Work out the finished part from the listing and answer in its coordinate system (mm). Give positions to 0.01 mm unless a question says otherwise; leave off trailing zeros. Order: outer loops, then holes, each group sorted by start corner. A loop starts at its lowest first (then second) coordinate and runs counter-clockwise, first axis right, second up. Notation, with made-up numbers: (-6.75, 71) - (9.25, 71) arc R17 cw to (9.25, 86) - close; hole circle Ø11 at (61.5, 40). An arc over 180 degrees is marked (long way). Return JSON: item names as keys, results as strings. Group by question number.
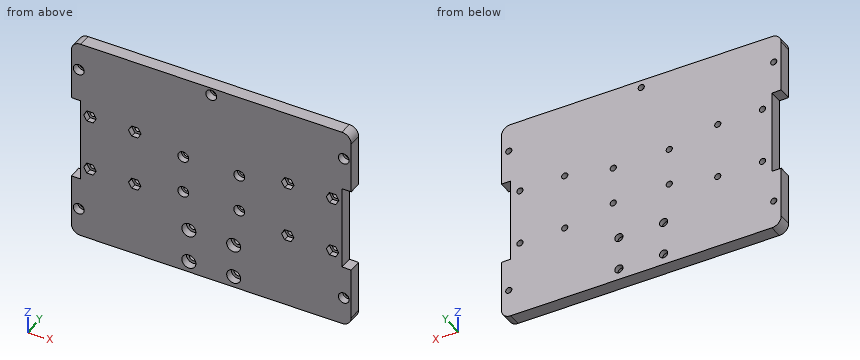
from build123d import *

# Parameters (mm, degrees)
SKETCH_1_W          = 150
SKETCH_1_H          = 110
EXTRUDE_1_DEPTH     = 7
FILLET_1_R          = 5
SKETCH_2_R          = 1.65
SKETCH_2_R_2        = 2.2
CUT_EXTRUDE_1_DEPTH = 8
SKETCH_5_R          = 3.75
CUT_EXTRUDE_3_DEPTH = 4.2
CUT_EXTRUDE_4_DEPTH = 3
SKETCH_7_R          = 2.9
CUT_EXTRUDE_5_DEPTH = 3.3
SKETCH_8_R          = 1.65
CUT_EXTRUDE_6_DEPTH = 8
SKETCH_9_R          = 2.9
CUT_EXTRUDE_7_DEPTH = 4
SKETCH_10_W         = 5
SKETCH_10_H         = 45
CUT_EXTRUDE_8_DEPTH = 8


with BuildPart() as part:
    # 草图1 → 凸台-拉伸1 (new body)
    with BuildSketch(Plane(origin=(0, 0, 0), x_dir=(1, 0, 0), z_dir=(0, 1, 0))):
        Rectangle(SKETCH_1_W, SKETCH_1_H)
    extrude(amount=EXTRUDE_1_DEPTH)

    # 圆角1
    fillet_1_edges = [part.edges().sort_by_distance(p)[0] for p in [
        (75, 3.5, 55),
        (-75, 3.5, 55),
        (-75, 3.5, -55),
        (75, 3.5, -55),
    ]]
    fillet(fillet_1_edges, radius=FILLET_1_R)

    # 草图2 → 切除-拉伸1 (cut, through all)
    with BuildSketch(Plane(origin=(0, 7, 0), x_dir=(1, 0, 0), z_dir=(0, 1, 0))):
        with Locations((65, -15)):
            Circle(SKETCH_2_R)
        with Locations((41, -15)):
            Circle(SKETCH_2_R)
        with Locations((41, 15)):
            Circle(SKETCH_2_R)
        with Locations((65, 15)):
            Circle(SKETCH_2_R)
        with Locations((-65, 15)):
            Circle(SKETCH_2_R)
        with Locations((-41, 15)):
            Circle(SKETCH_2_R)
        with Locations((-41, -15)):
            Circle(SKETCH_2_R)
        with Locations((-65, -15)):
            Circle(SKETCH_2_R)
        with Locations((12, 31)):
            Circle(SKETCH_2_R_2)
        with Locations((12, 49)):
            Circle(SKETCH_2_R_2)
        with Locations((-12, 49)):
            Circle(SKETCH_2_R_2)
        with Locations((-12, 31)):
            Circle(SKETCH_2_R_2)
        with Locations((15, 10)):
            Circle(SKETCH_2_R)
        with Locations((15, -10)):
            Circle(SKETCH_2_R)
        with Locations((-15, -10)):
            Circle(SKETCH_2_R)
        with Locations((-15, 10)):
            Circle(SKETCH_2_R)
    extrude(amount=-CUT_EXTRUDE_1_DEPTH, mode=Mode.SUBTRACT)

    # 草图5 → 切除-拉伸3 (cut)
    with BuildSketch(Plane.XZ):
        with Locations((12, -49)):
            Circle(SKETCH_5_R)
        with Locations((12, -31)):
            Circle(SKETCH_5_R)
        with Locations((-12, -31)):
            Circle(SKETCH_5_R)
        with Locations((-12, -49)):
            Circle(SKETCH_5_R)
    extrude(amount=-CUT_EXTRUDE_3_DEPTH, mode=Mode.SUBTRACT)

    # 草图6 → 切除-拉伸4 (cut)
    with BuildSketch(Plane.XZ):
        Polygon((-39.325684219, 17.9), (-37.651368439, 15), (-39.325684219, 12.1), (-42.674315781, 12.1), (-44.348631561, 15), (-42.674315781, 17.9), align=None)
        Polygon((61.651368439, -15), (63.325684219, -17.9), (66.674315781, -17.9), (68.348631561, -15), (66.674315781, -12.1), (63.325684219, -12.1), align=None)
        Polygon((37.651368439, -15), (39.325684219, -17.9), (42.674315781, -17.9), (44.348631561, -15), (42.674315781, -12.1), (39.325684219, -12.1), align=None)
        Polygon((61.651368439, 15), (63.325684219, 12.1), (66.674315781, 12.1), (68.348631561, 15), (66.674315781, 17.9), (63.325684219, 17.9), align=None)
        Polygon((37.651368439, 15), (39.325684219, 12.1), (42.674315781, 12.1), (44.348631561, 15), (42.674315781, 17.9), (39.325684219, 17.9), align=None)
        Polygon((-63.325684219, 17.9), (-61.651368439, 15), (-63.325684219, 12.1), (-66.674315781, 12.1), (-68.348631561, 15), (-66.674315781, 17.9), align=None)
        Polygon((-39.325684219, -12.1), (-37.651368439, -15), (-39.325684219, -17.9), (-42.674315781, -17.9), (-44.348631561, -15), (-42.674315781, -12.1), align=None)
        Polygon((-63.325684219, -12.1), (-61.651368439, -15), (-63.325684219, -17.9), (-66.674315781, -17.9), (-68.348631561, -15), (-66.674315781, -12.1), align=None)
    extrude(amount=-CUT_EXTRUDE_4_DEPTH, mode=Mode.SUBTRACT)

    # 草图7 → 切除-拉伸5 (cut)
    with BuildSketch(Plane.XZ):
        with Locations((15, -10)):
            Circle(SKETCH_7_R)
        with Locations((15, 10)):
            Circle(SKETCH_7_R)
        with Locations((-15, 10)):
            Circle(SKETCH_7_R)
        with Locations((-15, -10)):
            Circle(SKETCH_7_R)
    extrude(amount=-CUT_EXTRUDE_5_DEPTH, mode=Mode.SUBTRACT)

    # 草图8 → 切除-拉伸6 (cut, through all)
    with BuildSketch(Plane.XZ):
        with Locations((71, 40)):
            Circle(SKETCH_8_R)
        with Locations((71, -40)):
            Circle(SKETCH_8_R)
        with Locations((-71, -40)):
            Circle(SKETCH_8_R)
        with Locations((-71, 40)):
            Circle(SKETCH_8_R)
        with Locations((0, 51)):
            Circle(SKETCH_8_R)
    extrude(amount=-CUT_EXTRUDE_6_DEPTH, mode=Mode.SUBTRACT)

    # 草图9 → 切除-拉伸7 (cut)
    with BuildSketch(Plane.XZ):
        with Locations((71, 40)):
            Circle(SKETCH_9_R)
        with Locations((71, -40)):
            Circle(SKETCH_9_R)
        with Locations((-71, 40)):
            Circle(SKETCH_9_R)
        with Locations((-71, -40)):
            Circle(SKETCH_9_R)
        with Locations((0, 51)):
            Circle(SKETCH_9_R)
    extrude(amount=-CUT_EXTRUDE_7_DEPTH, mode=Mode.SUBTRACT)

    # 草图10 → 切除-拉伸8 (cut, through all)
    with BuildSketch(Plane(origin=(0, 7, 0), x_dir=(1, 0, 0), z_dir=(0, 1, 0))):
        with Locations((72.5, 0)):
            Rectangle(SKETCH_10_W, SKETCH_10_H)
        with Locations((-72.5, 0)):
            Rectangle(SKETCH_10_W, SKETCH_10_H)
    extrude(amount=-CUT_EXTRUDE_8_DEPTH, mode=Mode.SUBTRACT)


solid = part.part
1. The part is cut by section B-B (x = 0). Give the vertices of the cut face in (y, z), and give its area (3 significant figures).
2. The part is cut by section C-C (y = 1.5). State how many separate pieces and enclosed holes the cut face has, and give its area (3 significant figures).
3. The part is cut by section A-A (x = 41). Give the vertices of the cut face in (y, z), and give its area (3 significant figures).
4. Consider probe 1 along Z at (x, y) = (-64.5, 1.75); probe 2 along X at (y, z) = (5.75, -31); probe 3 along Z at (x, y) = (-12, 5.95). Determine where each line is inside the solid, lowest interval first. Write a range as from..to.
5. Each of these flat-tipped pins is pushed along its axis until it touches: pin 1 (6 mm diameter, centred on x = 12, z = -49, fed in from -Y); pin 2 (4.5 mm diameter, centred on x = 65.5, z = -15, fed in from -Y); pin 3 (3.5 mm diameter, centred on x = 71, z = 40, fed in from -Y). Where does it stop, or does it pass through?
Answers:
{
 "1": {"outline": "(0, -55) - (7, -55) - (7, 49.35) - (4, 49.35) - (4, 48.1) - (0, 48.1) - close; (0, 53.9) - (4, 53.9) - (4, 52.65) - (7, 52.65) - (7, 55) - (0, 55) - close", "area": "737 mm^2"},
 "2": {"separate pieces": "1", "enclosed holes": "21", "area": "15,400 mm^2"},
 "3": {"outline": "(0, -55) - (7, -55) - (7, -16.65) - (3, -16.65) - (3, -17.9) - (0, -17.9) - close; (0, -12.1) - (3, -12.1) - (3, -13.35) - (7, -13.35) - (7, 13.35) - (3, 13.35) - (3, 12.1) - (0, 12.1) - close; (0, 17.9) - (3, 17.9) - (3, 16.65) - (7, 16.65) - (7, 55) - (0, 55) - close", "area": "709 mm^2"},
 "4": {"probe 1": "z = -55..-17.9, -12.1..12.1, 17.9..55", "probe 2": "x = -75..-14.2, -9.8..9.8, 14.2..75", "probe 3": "z = -55..-51.2, -46.8..-33.2, -28.8..55"},
 "5": {"pin 1": "stops at y = 4.2", "pin 2": "stops at y = 3", "pin 3": "stops at y = 4"}
}
